Geometry check sheet. Reference: the model listing, model coordinates, mm. Give positions to 0.01 mm unless a question says otherwise; leave off trailing zeros. Order: outer loops, then holes, each group sorted by start corner. A loop starts at its lowest first (then second) coordinate and runs counter-clockwise, first axis right, second up. Notation, with made-up numbers: (47.5, 48.25) - (58.5, 48.25) arc R18 ccw to (58.5, 62.25) - close; hole circle Ø6 at (-33, -16.5). An arc over 180 degrees is marked (long way). Put each result on its own line as item: value. Start each with the question number.
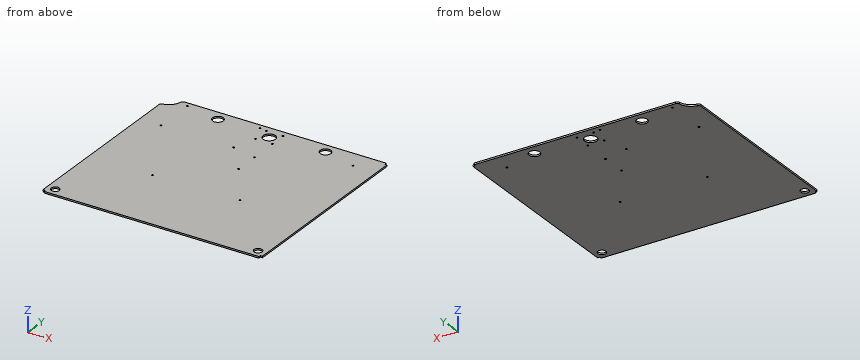
```python
from build123d import *

# Parameters (mm, degrees)
F0_R     = 7.5
F0_R_2   = 1.6
F0_R_3   = 10
F0_R_4   = 11.5
F1_DEPTH = 3


with BuildPart() as f1:
    # F0 (on Top) → F1 (new body)
    with BuildSketch(Plane.XY):
        with BuildLine():
            Line((90.722883, 364.83956), (-284.089221, 364.83956))
            ThreePointArc((-284.089221, 364.83956), (-287.307803, 363.665882), (-289.015352, 360.695854))
            ThreePointArc((-289.015352, 360.695854), (-295.88796, 347.463485), (-309.127945, 340.605561))
            ThreePointArc((-309.127945, 340.605561), (-312.101652, 338.899187), (-313.277117, 335.678484))
            Line((-313.277117, 335.678484), (-313.277117, 0.83956))
            Line((-313.277117, 0.83956), (-309.277117, 0.83956))
            Line((-309.277117, 0.83956), (-309.277117, -3.16044))
            Line((-309.277117, -3.16044), (90.722883, -3.16044))
            Line((90.722883, -3.16044), (90.722883, 0.83956))
            Line((90.722883, 0.83956), (94.722883, 0.83956))
            Line((94.722883, 0.83956), (94.722883, 360.83956))
            Line((94.722883, 360.83956), (90.722883, 360.83956))
            Line((90.722883, 360.83956), (90.722883, 364.83956))
        make_face()
        with Locations((-297.777117, 12.33956)):
            Circle(F0_R, mode=Mode.SUBTRACT)
        with Locations((-194.936931, 133.696496)):
            Circle(F0_R_2, mode=Mode.SUBTRACT)
        with Locations((79.222883, 12.33956)):
            Circle(F0_R, mode=Mode.SUBTRACT)
        with Locations((-35.277117, 137.83956)):
            Circle(F0_R_2, mode=Mode.SUBTRACT)
        with Locations((-273.277117, 279.83956)):
            Circle(F0_R_2, mode=Mode.SUBTRACT)
        with Locations((-273.277117, 355.83956)):
            Circle(F0_R_2, mode=Mode.SUBTRACT)
        with Locations((-138.277117, 279.83956)):
            Circle(F0_R_2, mode=Mode.SUBTRACT)
        with Locations((-209.277117, 344.83956)):
            Circle(F0_R_3, mode=Mode.SUBTRACT)
        with Locations((-124.777117, 322.33956)):
            Circle(F0_R_2, mode=Mode.SUBTRACT)
        with Locations((-138.277117, 355.83956)):
            Circle(F0_R_2, mode=Mode.SUBTRACT)
        with Locations((-124.777117, 353.33956)):
            Circle(F0_R_2, mode=Mode.SUBTRACT)
        with Locations((-93.068697, 223.877582)):
            Circle(F0_R_2, mode=Mode.SUBTRACT)
        with Locations((-93.068697, 269.877582)):
            Circle(F0_R_2, mode=Mode.SUBTRACT)
        with Locations((-93.777117, 322.33956)):
            Circle(F0_R_2, mode=Mode.SUBTRACT)
        with Locations((-109.277117, 337.83956)):
            Circle(F0_R_4, mode=Mode.SUBTRACT)
        with Locations((-93.777117, 353.33956)):
            Circle(F0_R_2, mode=Mode.SUBTRACT)
        with Locations((-9.277117, 344.83956)):
            Circle(F0_R_3, mode=Mode.SUBTRACT)
        with Locations((51.722883, 329.83956)):
            Circle(F0_R_2, mode=Mode.SUBTRACT)
    extrude(amount=F1_DEPTH)


solid = f1.part
```
Item 1: Gauge pin test, flat ends, axial feed: pin 1 Ø1.5 at (y, z) = (-1.5, 1) entering from -X; pin 2 Ø0.9 at (y, z) = (363.5, 1.5) entering from +X; pin 3 Ø0.9 at (x, z) = (92, 2) entering from +Y. Record the tip position at first contact, or that the pin passes through.
Item 2: Cross-section at A-A (x = -210.5). Enter the section's corners in (y, z).
Item 3: Thickness scan on line 1 along Y through (x, z) = (-293, 0.7); line 2 along Y through (x, z) = (53, 1.65). Record the ranges inside material, lowest first.
Item 4: Cross-section at B-B (x = -5). Enter the section's corners in (y, z), and give its area (3 significant figures).
Recorded:
1. pin 1: stops at x = -309.28
1. pin 2: stops at x = 90.72
1. pin 3: stops at y = 360.84
2. outline: (-3.16, 0) - (334.91, 0) - (334.91, 3) - (-3.16, 3) - close; (354.76, 0) - (364.84, 0) - (364.84, 3) - (354.76, 3) - close
3. line 1: y = -3.16 to 6.56, 18.12 to 350.93
3. line 2: y = -3.16 to 328.88, 330.8 to 364.84
4. outline: (-3.16, 0) - (335.8, 0) - (335.8, 3) - (-3.16, 3) - close; (353.88, 0) - (364.84, 0) - (364.84, 3) - (353.88, 3) - close
4. area: 1,050 mm^2
